Could you check a few things on this model? Use its own coordinates, in mm. A direction names the side the tool comes from. Give positions to 0.01 mm unless a question says otherwise; leave off trailing zeros. Loops run counter-clockwise (first coordinate to the right, second up) from the corner with the lowest first, then second, coordinate; pieces in that order, holes last. Notation, with made-up numbers: (23.25, 25.5) - (71.25, 25.5) arc R23 ccw to (71.25, 60.5) - close; hole circle Ø7 at (45.5, -25.5). An arc over 180 degrees is marked (long way). One line per item, written item: value. Start each with the question number.
Q1. If we mould it in two halves opening along Z, with no side actions, what happens to faces 5 (the face through (-14.3, 0, 21.3)), 6 (the face through (0, -25.4, 0)), 7 (the face through (0, 38.1, 0)), 8 (the face through (-6.883, -25.044, -30.995))? For each: released by +Z, released by -Z, zero draft, split by the parting line, or undercut.
Q2. For faces 1 (the face through (0, -76.2, 0)), 2 (the face through (7, -50.8, -7)), 3 (the face through (1.323, 125.755, 10.074)), 4 (the face through (-23.016, 125.755, 7.248)), which set-ups out of +Z, -Z, +X, -X, +Y, -Y let a thin tool reach every point of the face, with its end or its side?
Q3. I want a section at B-B (y = -31). Please give me the cut outline in (x, z).
Q4. I'm going to push flat-ended pins straight in: P1, Ø10, axis at x = 0, z = 0, coming from the +Y side; P2, Ø2, axis at x = 18, z = 13.5, coming from the +Y side; P3, Ø2, axis at y = 165, z = 8, coming from the -X side. Where does each tip first touch, or does it pass through?
Q5. If I drill on line 1 (Z direction, x = 0, y = 82); line 2 (Z direction, x = 0, y = -19.5); line 3 (Y direction, x = -27.5, z = -5), over which ranges is the centre line in solid material (lowest first)? Write a range as from..to.
Q6. I want a section at A-A (y = 69.5). Please give me the cut outline in (x, z), then the cut area to 3 significant figures.
```python
from build123d import *

# Parameters (mm, degrees)
F1_R      = 6.35
F2_DEPTH  = 5.842
F3_R      = 6.35
F4_DEPTH  = 2.54
F5_R      = 31.75
F5_R_2    = 6.35
F6_DEPTH  = 50.8
F7_R      = 7.62
F7_R_2    = 6.35
F8_DEPTH  = 25.4
F9_R      = 6.35
F12_R     = 25.4
F13_DEPTH = 38.1
F14_R     = 35.052
F14_R_2   = 22.86
F15_DEPTH = 5.842
F16_SIZE2 = 6.9785926454
F16_SIZE  = 2.54
F17_R     = 28.0734073546
F17_R_2   = 24.13
F18_DEPTH = 2.54
F19_R     = 26.8034073546
F19_R_2   = 24.13
F20_DEPTH = 2.54
F21_R     = 24.1300254
F21_R_2   = 10.16
F22_DEPTH = 177.8
F23_R     = 10.668
F23_R_2   = 7.874
F24_DEPTH = 50.8


with BuildPart() as f2:
    # F1 (on Front) → F2 (new body)
    with BuildSketch(Plane.XZ):
        Circle(F1_R)
    extrude(amount=-F2_DEPTH)

    # F3 (on face) → F4 (join)
    with BuildSketch(Plane(origin=(0, 5.842, 0), x_dir=(-1, 0, 0), z_dir=(0, 1, 0))):
        Circle(F3_R)
    extrude(amount=F4_DEPTH)

    # F5 (on face) → F6 (join)
    with BuildSketch(Plane.XZ):
        Circle(F5_R)
        Circle(F5_R_2, mode=Mode.SUBTRACT)
    extrude(amount=F6_DEPTH)

    # F7 (on face) → F8 (join)
    with BuildSketch(Plane.XZ.offset(50.8)):
        Circle(F7_R)
        Circle(F7_R_2, mode=Mode.SUBTRACT)
    extrude(amount=F8_DEPTH)

    # F11: sweep along a path in F10
    with BuildLine(Plane.YZ) as f11_path:
        Line((-76.2, 0), (-25.4, 0))
    # F9 (on face) → F11 (sweep)
    with BuildSketch(Plane.XZ.offset(76.2)):
        Circle(F9_R)
    sweep(path=f11_path.line)

    # F12 (on face) → F13 (join)
    with BuildSketch(Plane(origin=(0, 0, 0), x_dir=(-1, 0, 0), z_dir=(0, 1, 0))):
        Circle(F12_R)
    extrude(amount=F13_DEPTH)

    # F14 (on face) → F15 (join)
    with BuildSketch(Plane(origin=(0, 38.1, 0), x_dir=(-1, 0, 0), z_dir=(0, 1, 0))):
        Circle(F14_R)
        Circle(F14_R_2, mode=Mode.SUBTRACT)
    extrude(amount=-F15_DEPTH)

    # F16
    f16_edges = [f2.edges().sort_by_distance(p)[0] for p in [
        (35.052, 32.258, 0),
    ]]
    f16_side = f2.faces().sort_by_distance((35.052, 35.179, 0))[0]
    chamfer(f16_edges, length=F16_SIZE, length2=F16_SIZE2, reference=f16_side)

    # F17 (on face) → F18 (join)
    with BuildSketch(Plane.XZ.offset(-32.258)):
        Circle(F17_R)
        Circle(F17_R_2, mode=Mode.SUBTRACT)
    extrude(amount=F18_DEPTH)

    # F19 (on face) → F20 (join)
    with BuildSketch(Plane.XZ.offset(-29.718)):
        Circle(F19_R)
        Circle(F19_R_2, mode=Mode.SUBTRACT)
    extrude(amount=F20_DEPTH)

    # F21 (on face) → F22 (join)
    with BuildSketch(Plane(origin=(0, 38.1, 0), x_dir=(-1, 0, 0), z_dir=(0, 1, 0))):
        Circle(F21_R)
        Circle(F21_R_2, mode=Mode.SUBTRACT)
    extrude(amount=F22_DEPTH)

    # F23 (on face) → F24 (join)
    with BuildSketch(Plane(origin=(0, 215.9, 0), x_dir=(-1, 0, 0), z_dir=(0, 1, 0))):
        Circle(F23_R)
        Circle(F23_R_2, mode=Mode.SUBTRACT)
    extrude(amount=F24_DEPTH)


solid = f2.part
```
Worked answers:
1. face 5: zero draft
1. face 6: undercut
1. face 7: undercut
1. face 8: split by the parting line
2. face 1: +Z, -Z, +X, -X, -Y
2. face 2: -Y
2. face 3: none
2. face 4: +Y
3. outline: circle Ø63.5 at (0, 0)
4. P1: stops at y = 38.1
4. P2: stops at y = 215.9
4. P3: stops at x = -23.09
5. line 1: z = -24.13..-10.16, 10.16..24.13
5. line 2: z = -31.75..-6.35, 6.35..31.75
5. line 3: y = -50.8..0, 29.72..38.1
6. outline: circle Ø48.26 at (0, 0); hole circle Ø20.32 at (0, 0)
6. area: 1,500 mm²
